Verification items for the finished model (mm, model axes). Round coordinates to 2 decimals unless told otherwise and drop trailing zeros. Write each loop counter-clockwise with the first axis right and the second up, starting at its lowest first coordinate (ties: lowest second). Pieces come first, ordered by that corner, then holes. Notation, with made-up numbers: M 77.25,35 L 123.25,35 A22 ccw 123.25,66 Z; hole C 83.25,14.25 d8. An arc over 180 degrees is marked long. One line per item, written item: value. Start each with the question number.
Item 1: Section check A-A, the plane z = 2.1. State how many separate pieces and enclosed holes the cut face has, then the cut area to 3 significant figures.
Item 2: Thickness scan on probe 1 along Y at (x, z) = (-401.75, 2.1); probe 2 along X at (y, z) = (97, 0.35). Record the ranges inside material, lowest first. Write a range as from..to.
Item 3: Gauge pin test, flat ends, axial feed: pin 1 (3.5 mm diameter, centred on x = -5.75, y = 23.62, fed in from -Z); pin 2 (1 mm diameter, centred on y = 173, z = 3, fed in from -X); pin 3 (2 mm diameter, centred on y = 273.5, z = 3, fed in from +X). Record the tip position at first contact, or that the pin passes through.
Item 4: Section check B-B, the plane y = 89. Record the cut outline in (x, z), then the cut area to 3 significant figures.
Autodesk Inventor part; units mm, degrees
ref_plane "YZ Plane" through (0, 0, 0) normal (1, 0, 0) x (0, 1, 0)
ref_plane "XZ Plane" through (0, 0, 0) normal (0, 1, 0) x (-1, 0, 0)
ref_plane "XY Plane" through (0, 0, 0) normal (0, 0, 1) x (1, 0, 0)
ref_plane "Work Plane1" through (0, 10, 0) normal (0, 0, 1) x (1, 0, 0)
sketch "Sketch1" plane through (0, 10, 0) normal (0, 0, 1) x (1, 0, 0)
  line L0 (-1, 70.8708) -> (-1, -7.0974)
  line L1 (-1, 70.8708) -> (-53.0809, 70.8708)
  arc A0 (-53.0809, 70.8708) -> (-59.8755, 68.2079) centre (-53.0809, 60.8708) ccw
  line L2 (-59.8755, 68.2079) -> (-118.9152, 13.5337)
  line L3 (-1, -7.0974) -> (-454, -7.0974)
  circle A1 centre (-53.25, 13.6208) radius 2.067
  circle A2 centre (-53.25, 61.1208) radius 2.067
  circle A3 centre (-5.75, 13.6208) radius 2.067
  circle A4 centre (-5.75, 61.1208) radius 2.067
  circle A5 centre (-401.75, 61.1208) radius 2.067
  circle A6 centre (-449.25, 61.1208) radius 2.067
  circle A7 centre (-401.75, 13.6208) radius 2.067
  circle A8 centre (-449.25, 13.6208) radius 2.067
  line L4 (-454, -7.0974) -> (-454, 70.8708)
  line L5 (-1, -7.0974) -> (-454, -7.0974)
  arc A9 (-344.754, 14.034) -> (-337.4562, 10.8708) centre (-337.4562, 20.8708) ccw
  line L6 (-344.754, 14.034) -> (-395.0366, 67.7076)
  arc A10 (-395.0366, 67.7076) -> (-402.3345, 70.8708) centre (-402.3345, 60.8708) ccw
  line L7 (-402.3345, 70.8708) -> (-454, 70.8708)
  arc A11 (-436.1083, -78.4697) -> (-447.5, -37.6782) centre (-447.5, -59.6646) ccw
  line L8 (-18.8917, -78.4697) -> (-436.1083, -78.4697)
  arc A12 (-7.5, -37.6782) -> (-18.8917, -78.4697) centre (-7.5, -59.6646) ccw
  line L9 (-2, -37.6782) -> (-7.5, -37.6782)
  arc A13 (-2, -37.6782) -> (-1, -36.6782) centre (-2, -36.6782) ccw
  line L10 (-1, -12.4515) -> (-1, -36.6782)
  line L11 (-454, -12.4515) -> (-1, -12.4515)
  line L12 (-454, -36.6782) -> (-454, -12.4515)
  arc A14 (-454, -36.6782) -> (-453, -37.6782) centre (-453, -36.6782) ccw
  line L13 (-447.5, -37.6782) -> (-453, -37.6782)
  line L14 (-237.5, -48.429) -> (-237.5, -34.9155)
  ellipse E0 centre (-235.5, -34.9155) end of major axis (-237.5, -34.9155) minor radius 1.6892 (-235.5, -33.2263) -> (-237.5, -34.9155) ccw
  line L15 (-235.5, -33.2263) -> (-219.5, -33.2263)
  ellipse E1 centre (-219.5, -34.9155) end of major axis (-221.5, -34.9155) minor radius 1.6892 (-217.5, -34.9155) -> (-219.5, -33.2263) ccw
  line L16 (-217.5, -34.9155) -> (-217.5, -48.429)
  ellipse E2 centre (-219.5, -48.429) end of major axis (-217.5, -48.429) minor radius 1.6892 (-219.5, -50.1182) -> (-217.5, -48.429) ccw
  line L17 (-219.5, -50.1182) -> (-235.5, -50.1182)
  ellipse E3 centre (-235.5, -48.429) end of major axis (-233.5, -48.429) minor radius 1.6892 (-237.5, -48.429) -> (-235.5, -50.1182) ccw
  line L18 (-267.5, -48.429) -> (-267.5, -34.9155)
  ellipse E4 centre (-265.5, -34.9155) end of major axis (-267.5, -34.9155) minor radius 1.6892 (-265.5, -33.2263) -> (-267.5, -34.9155) ccw
  line L19 (-265.5, -33.2263) -> (-249.5, -33.2263)
  ellipse E5 centre (-249.5, -34.9155) end of major axis (-251.5, -34.9155) minor radius 1.6892 (-247.5, -34.9155) -> (-249.5, -33.2263) ccw
  line L20 (-247.5, -34.9155) -> (-247.5, -48.429)
  ellipse E6 centre (-249.5, -48.429) end of major axis (-247.5, -48.429) minor radius 1.6892 (-249.5, -50.1182) -> (-247.5, -48.429) ccw
  line L21 (-249.5, -50.1182) -> (-265.5, -50.1182)
  ellipse E7 centre (-265.5, -48.429) end of major axis (-263.5, -48.429) minor radius 1.6892 (-267.5, -48.429) -> (-265.5, -50.1182) ccw
  line L22 (-205.5, -33.2263) -> (-189.5, -33.2263)
  ellipse E8 centre (-189.5, -34.9155) end of major axis (-191.5, -34.9155) minor radius 1.6892 (-187.5, -34.9155) -> (-189.5, -33.2263) ccw
  line L23 (-187.5, -34.9155) -> (-187.5, -48.429)
  ellipse E9 centre (-189.5, -48.429) end of major axis (-187.5, -48.429) minor radius 1.6892 (-189.5, -50.1182) -> (-187.5, -48.429) ccw
  line L24 (-189.5, -50.1182) -> (-205.5, -50.1182)
  ellipse E10 centre (-205.5, -48.429) end of major axis (-203.5, -48.429) minor radius 1.6892 (-207.5, -48.429) -> (-205.5, -50.1182) ccw
  line L25 (-207.5, -48.429) -> (-207.5, -34.9155)
  ellipse E11 centre (-205.5, -34.9155) end of major axis (-207.5, -34.9155) minor radius 1.6892 (-205.5, -33.2263) -> (-207.5, -34.9155) ccw
  line L26 (-395, -52.2297) -> (-395, -31.1148)
  ellipse E12 centre (-385, -31.1148) end of major axis (-395, -31.1148) minor radius 8.4459 (-385, -22.6689) -> (-395, -31.1148) ccw
  line L27 (-385, -22.6689) -> (-310, -22.6689)
  ellipse E13 centre (-310, -31.1148) end of major axis (-320, -31.1148) minor radius 8.4459 (-300, -31.1148) -> (-310, -22.6689) ccw
  line L28 (-300, -31.1148) -> (-300, -52.2297)
  ellipse E14 centre (-310, -52.2297) end of major axis (-300, -52.2297) minor radius 8.4459 (-310, -60.6756) -> (-300, -52.2297) ccw
  line L29 (-310, -60.6756) -> (-385, -60.6756)
  ellipse E15 centre (-385, -52.2297) end of major axis (-375, -52.2297) minor radius 8.4459 (-395, -52.2297) -> (-385, -60.6756) ccw
  line L30 (-145, -22.6689) -> (-70, -22.6689)
  ellipse E16 centre (-70, -31.1148) end of major axis (-80, -31.1148) minor radius 8.4459 (-60, -31.1148) -> (-70, -22.6689) ccw
  line L31 (-60, -31.1148) -> (-60, -52.2297)
  ellipse E17 centre (-70, -52.2297) end of major axis (-60, -52.2297) minor radius 8.4459 (-70, -60.6756) -> (-60, -52.2297) ccw
  line L32 (-70, -60.6756) -> (-145, -60.6756)
  ellipse E18 centre (-145, -52.2297) end of major axis (-135, -52.2297) minor radius 8.4459 (-155, -52.2297) -> (-145, -60.6756) ccw
  line L33 (-155, -52.2297) -> (-155, -31.1148)
  ellipse E19 centre (-145, -31.1148) end of major axis (-155, -31.1148) minor radius 8.4459 (-145, -22.6689) -> (-155, -31.1148) ccw
  circle A15 centre (-53.25, 13.6208) radius 2.067
  circle A16 centre (-53.25, 61.1208) radius 2.067
  circle A17 centre (-5.75, 13.6208) radius 2.067
  circle A18 centre (-5.75, 61.1208) radius 2.067
  line L34 (-1, 70.8708) -> (-1, -7.0974)
  line L35 (-1, 70.8708) -> (-53.0809, 70.8708)
  arc A19 (-53.0809, 70.8708) -> (-59.8755, 68.2079) centre (-53.0809, 60.8708) ccw
  line L36 (-59.8755, 68.2079) -> (-118.9152, 13.5337)
  arc A20 (-125.7098, 10.8708) -> (-118.9152, 13.5337) centre (-125.7098, 20.8708) ccw
  line L37 (-125.7098, 10.8708) -> (-337.4562, 10.8708)
  circle A21 centre (-449.25, 13.6208) radius 2.067
  circle A22 centre (-401.75, 13.6208) radius 2.067
  circle A23 centre (-449.25, 61.1208) radius 2.067
  circle A24 centre (-401.75, 61.1208) radius 2.067
  line L38 (-454, -7.0974) -> (-454, 70.8708)
  arc A25 (-125.7098, 10.8708) -> (-118.9152, 13.5337) centre (-125.7098, 20.8708) ccw
  line L39 (-125.7098, 10.8708) -> (-337.4562, 10.8708)
  arc A26 (-344.754, 14.034) -> (-337.4562, 10.8708) centre (-337.4562, 20.8708) ccw
  line L40 (-344.754, 14.034) -> (-395.0366, 67.7076)
  arc A27 (-395.0366, 67.7076) -> (-402.3345, 70.8708) centre (-402.3345, 60.8708) ccw
  line L41 (-402.3345, 70.8708) -> (-454, 70.8708)
  circle A28 centre (-227.5, 1.8867) radius 4
  line L42 (-227.5, 1.8867) -> (-227.5, -7.0974) construction
  line L43 (-227.5, 1.8867) -> (-227.5, 10.8708) construction
  line L44 (51.5, 217.3708) -> (43.5, 217.3708)
  line L45 (-506.5, 217.3708) -> (-498.5, 217.3708)
  line L46 (-1, -7.0974) -> (-454, -7.0974)
  line L47 (-455, 417.3708) -> (0, 417.3708)
  line L48 (-455, 70.8708) -> (-455, 6.8872)
  line L49 (0, -7.0974) -> (0, 70.8708)
  line L50 (-455, -7.0974) -> (-455, 417.3708)
  line L51 (0, -7.0974) -> (0, 417.3708)
  line L52 (-1, -7.0974) -> (0, -7.0974)
  line L53 (-454, -7.0974) -> (-455, -7.0974)
  point P0 (0, -10)
  point P1 (-227.5, -33.2263)
  point P2 (0, 70.8708)
  point P3 (-455, 6.8872)
  point P4 (-454, -7.0974)
  dimension "d0" = 8
  dimension "d1" = 200
extrude "Extrusion1" add sketch "Sketch1" along normal blind 4 contours L1 A0 L2 A20 L37 A9 L6 A10 L7 L4 L53 L50 L48 L47 L51 L49 L52 L0 | L0 L3 L4 L7 A10 L6 A9 L37 A20 L2 A0 L1
sketch "Sketch2" plane through (0, 10, 4) normal (0, 0, 1) x (1, 0, 0)
  line L0 (0, -7.0974) -> (0, 417.3708)
  line L1 (0, 417.3708) -> (-455, 417.3708)
  line L2 (-455, 417.3708) -> (-455, -7.0974)
  line L3 (-455, -7.0974) -> (0, -7.0974)
  circle A0 centre (-227.5, 1.8867) radius 4
  circle A1 centre (-449.25, 13.6208) radius 2.067
  circle A2 centre (-53.25, 13.6208) radius 2.067
  circle A3 centre (-53.25, 61.1208) radius 2.067
  circle A4 centre (-5.75, 13.6208) radius 2.067
  circle A5 centre (-5.75, 61.1208) radius 2.067
  circle A6 centre (-401.75, 61.1208) radius 2.067
  circle A7 centre (-449.25, 61.1208) radius 2.067
  circle A8 centre (-401.75, 13.6208) radius 2.067
  line L4 (-455, 417.3708) -> (-455, -7.0974)
  line L5 (0, -7.0974) -> (-455, -7.0974)
  line L6 (-455, -7.0974) -> (-455, 5.8867)
  line L7 (-455, 5.8867) -> (0, 5.8867)
  line L8 (0, 5.8867) -> (0, -7.0974)
  point P0 (0, -10)
extrude "Cut1" cut sketch "Sketch2" against normal up to next contours L3 L2 L7 L0
sketch "Sketch3" plane through (0, 10, 0) normal (0, 0, -1) x (-1, 0, 0)
  circle A0 centre (401.75, 13.6208) radius 2.067
  circle A1 centre (449.25, 61.1208) radius 2.067
  circle A2 centre (401.75, 61.1208) radius 2.067
  circle A3 centre (5.75, 61.1208) radius 2.067
  circle A4 centre (5.75, 13.6208) radius 2.067
  circle A5 centre (53.25, 61.1208) radius 2.067
  circle A6 centre (53.25, 13.6208) radius 2.067
  circle A7 centre (449.25, 13.6208) radius 2.067
  line L0 (0, 5.8867) -> (455, 5.8867)
  line L1 (455, 417.3708) -> (455, 5.8867)
  line L2 (0, 417.3708) -> (455, 417.3708)
  line L3 (0, 5.8867) -> (0, 417.3708)
  line L4 (455, 417.3708) -> (450, 417.3708)
  line L5 (450, 417.3708) -> (450, 70.8708)
  line L6 (450, 70.8708) -> (455, 70.8708)
  line L7 (455, 70.8708) -> (455, 417.3708)
  line L8 (0, 417.3708) -> (5, 417.3708)
  line L9 (5, 417.3708) -> (5, 70.8708)
  line L10 (5, 70.8708) -> (0, 70.8708)
  line L11 (0, 70.8708) -> (0, 417.3708)
  point P0 (0, -10)
  dimension "d7" = 5
  dimension "d8" = 346.5
extrude "Cut2" cut sketch "Sketch3" against normal through all contours L3 L2 L9 L10 | L6 L5 L2 L1
equation "\"d5\" = Thickness"
equation "\"d9\" = Thickness"
equation "\"BendRadius\" = Thickness"
equation "\"BendReliefWidth\" = Thickness"
equation "\"BendReliefDepth\" = 0.5 * Thickness"
equation "\"CornerReliefSize\" = 4 * Thickness"
equation "\"MinimumRemnant\" = 2 * Thickness"
equation "\"TransitionRadius\" = BendRadius"
equation "\"JacobiRadiusSize\" = Thickness"
equation "\"GapSize\" = Thickness"
equation "\"d4\" = Thickness"
properties part number "voetensteun"
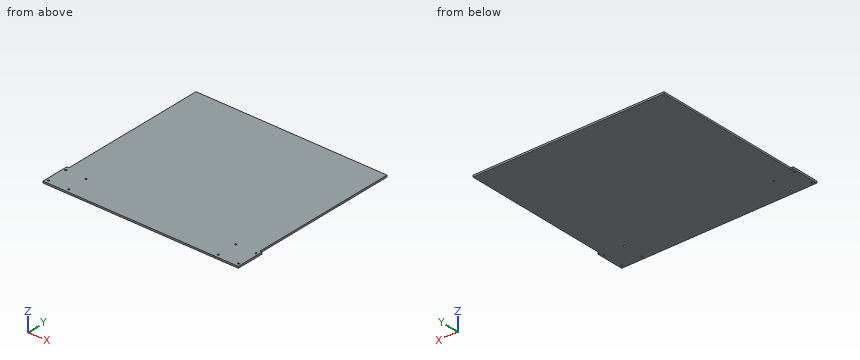
Response values:
1. separate pieces: 1
1. enclosed holes: 8
1. area: 184,000 mm2
2. probe 1: y = 15.89..21.55, 25.69..69.05, 73.19..427.37
2. probe 2: x = -450..-5
3. pin 1: passes through
3. pin 2: stops at x = -450
3. pin 3: stops at x = -5
4. outline: M -450,0 L -5,0 L -5,4 L -450,4 Z
4. area: 1,780 mm2
